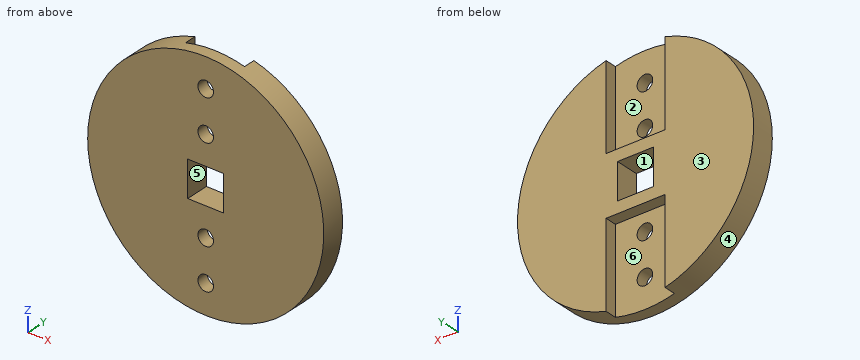
Autodesk Inventor part; units mm, degrees
ref_plane "Work Plane1" through (0, 0, 20) normal (0, 0, 1) x (1, 0, 0)
ref_plane "YZ Plane" through (0, 0, 0) normal (1, 0, 0) x (0, 1, 0)
ref_plane "XZ Plane" through (0, 0, 0) normal (0, 1, 0) x (-1, 0, 0)
sketch "Sketch1" plane through (0, 0, 0) normal (0, 1, 0) x (-1, 0, 0)
  circle A0 centre (0, 0) radius 20
  dimension "d0" = 40
extrude "Extrusion1" add sketch "Sketch1" along normal blind 6
sketch "Sketch3" plane through (0, 6, 0) normal (0, 1, 0) x (1, 0, 0)
  line L0 (0, 0) -> (0, 20)
  circle A0 centre (0, 0) radius 20
  line L1 (5, 35) -> (5, 5)
  line L2 (5, 5) -> (-5, 5)
  line L3 (-5, 5) -> (-5, 35)
  line L4 (-5, 35) -> (5, 35)
  line L5 (5, 35) -> (-5, 5) construction
  line L6 (5, 5) -> (-5, 35) construction
  line L7 (20, 0) -> (-20, 0) construction
  line L8 (5, -35) -> (5, -5)
  line L9 (5, -5) -> (-5, -5)
  line L10 (-5, -5) -> (-5, -35)
  line L11 (-5, -35) -> (5, -35)
  point P0 (-5, 19.3649)
  point P1 (5, 19.3649)
  point P2 (-5, -19.3649)
  point P3 (5, -19.3649)
  dimension "d11" = 30
  dimension "d12" = 10
extrude "Extrusion2" cut sketch "Sketch3" against normal blind 2 contours L2 L3 A0 L0 | L0 A0 L1 L2 | L10 L9 L8 A0
sketch "Sketch5" plane through (0, 4, 0) normal (0, 1, 0) x (1, 0, 0)
  circle A0 centre (0, -8) radius 1
  circle A1 centre (0, -15) radius 1
  line L0 (-5, -5) -> (5, -5)
  arc A2 (-5, 19.3649) -> (-5, -19.3649) centre (0, 0) ccw
  line L1 (-20, 0) -> (20, 0) construction
  arc A3 (5, -19.3649) -> (5, 19.3649) centre (0, 0) ccw
  circle A4 centre (0, 8) radius 1
  circle A5 centre (0, 15) radius 1
  line L2 (-28, 0) -> (28, 0)
  line L3 (-5, 5) -> (-5, 19.3649)
  dimension "d20" = 2
  dimension "d21" = 2
  dimension "d42" = 8
  dimension "d43" = 7
  dimension "d44" = 8
  dimension "d45" = 20
  dimension "d47" = 5
hole "Hole2" at (0, 4, 15) at (0, 4, 8) at (0, 4, -8) at (0, 4, -15) direction (0, -1, 0) diameter 2.6416 depth 10.979 tip angle 118
sketch "Sketch6" plane through (0, 6, 0) normal (0, 1, 0) x (1, 0, 0)
  line L0 (3.05, 3.05) -> (-3.05, 3.05)
  line L1 (-3.05, 3.05) -> (-3.05, -3.05)
  line L2 (-3.05, -3.05) -> (3.05, -3.05)
  line L3 (3.05, -3.05) -> (3.05, 3.05)
  point P0 (0, 0)
  dimension "d31" = 6.1
  dimension "d32" = 6.1
  dimension "d33" = 3.05
  dimension "d34" = 3.05
extrude "Extrusion4" cut sketch "Sketch6" against normal blind 10
ref_plane "Work Plane1" through (0, 0, 20) normal (0, 0, 1) x (1, 0, 0)
sketch "Sketch7" plane through (0, 0, 20) normal (0, 0, 1) x (1, 0, 0)
  line L0 (20, 0) -> (-20, 0)
  line L1 (-20, 0) -> (20, 0)
  line L2 (20, 0) -> (20, 2)
  line L3 (20, 2) -> (-20, 2)
  line L4 (-20, 2) -> (-20, 0)
  point P0 (0, 0)
  dimension "d38" = 40
  dimension "d39" = 2
extrude "Extrusion5" cut sketch "Sketch7" against normal blind 40
sketch "Sketch8" plane through (0, 6, 0) normal (0, 1, 0) x (1, 0, 0)
  line L0 (-20, -20) -> (-7, -20)
  line L1 (-7, -20) -> (-7, 20)
  line L2 (-7, 20) -> (-20, 20)
  line L3 (-20, 20) -> (-20, -20)
  line L4 (7, -20) -> (20, -20)
  line L5 (20, -20) -> (20, 20)
  line L6 (20, 20) -> (7, 20)
  line L7 (7, 20) -> (7, -20)
  line L8 (5, 19.3649) -> (5, 5)
  line L9 (-5, 5) -> (-5, 19.3649)
  line L10 (28.233, -20) -> (-28.0388, -20)
  point P0 (0, 0)
  dimension "d48" = 40
  dimension "d49" = 0
  dimension "d50" = 0
  dimension "d51" = 2
  dimension "d52" = 2
  dimension "d53" = 0
  dimension "d54" = 13
  dimension "d55" = 13
properties part number "prop_base"
Can you work these out from the model? Positions are in its coordinate system, mm. Face numbers are marked on the shaded views. A direction names the side the tool comes from. Round coordinates to 2 decimals unless told otherwise and drop trailing zeros. Loops run counter-clockwise (first coordinate to the right, second up) from the corner with the lowest first, then second, coordinate; pieces in that order, holes last. Notation, with made-up numbers: M 67.25,20 L 111.25,20 A22 cw 111.25,39 Z; hole C 24,67.25 d10. An arc over 180 degrees is marked long. Answer as a JSON object with one key per item and string values. Group by question number.
Q1. Will these pins go through, and if not, where does the flat tip stop? pin 1 (1 mm diameter, centred on y = 5.5, z = -3.5, fed in from -X); pin 2 (2 mm diameter, centred on y = 5.5, z = 14.5, fed in from +X); pin 3 (1 mm diameter, centred on y = 5, z = -10, fed in from +X); pin 4 (1.6 mm diameter, centred on x = 0, z = 8, fed in from +Y).
Q2. On a 3-axis mill with a long thin cutter (end or side, diameter ignored), from which of +Z, -Z, +X, -X, +Y, -Y can I reach the whole of each face in a straight line? I mean the marked faces 1, 2 and 3. Say none if no direction works.
Q3. We'd pull the mould along Z, two halves only. Please class the marked faces 4, 5 and 6: +Z half, -Z half, draft (parallel to the pull), parting line (faces both ways), or undercut.
Q4. Imagine slicing it at C-C, the plane x = 0. Please give me the cut outline in (y, z).
Q5. Imagine slicing it at B-B, the plane z = 0. Please give me the cut outline in (x, y), then the cut area to 3 significant figures.
Q6. Imagine slicing it at D-D, the plane z = -6. Please give me the cut outline in (x, y), then the cut area to 3 significant figures.
Q7. Imagine slicing it at A-A, the plane y = 4.7. Please give me the cut outline in (x, z), then the cut area to 3 significant figures.
Q8. Please list where these lines run through material, in increasing order: L1, parallel to Z at x = 0, y = 2.8; L2, parallel to Z at x = 0.5, y = 2.2; L3, parallel to X at y = 2.9, z = -8.
Findings:
{
 "1": {"pin 1": "stops at x = -19.77", "pin 2": "stops at x = 14.76", "pin 3": "stops at x = 17.6", "pin 4": "passes through"},
 "2": {"face 1": "+Y, -Y", "face 2": "+Z, +Y", "face 3": "+Z, -Z, +X, -X, +Y"},
 "3": {"face 4": "parting line", "face 5": "undercut", "face 6": "draft"},
 "4": {"outline": "M 2,-20 L 4,-20 L 4,-16.32 L 2,-16.32 Z; M 2,-13.68 L 4,-13.68 L 4,-9.32 L 2,-9.32 Z; M 2,-6.68 L 4,-6.68 L 4,-5 L 6,-5 L 6,-3.05 L 2,-3.05 Z; M 2,3.05 L 6,3.05 L 6,5 L 4,5 L 4,6.68 L 2,6.68 Z; M 2,9.32 L 4,9.32 L 4,13.68 L 2,13.68 Z; M 2,16.32 L 4,16.32 L 4,20 L 2,20 Z"},
 "5": {"outline": "M -20,2 L -3.05,2 L -3.05,6 L -20,6 Z; M 3.05,2 L 20,2 L 20,6 L 3.05,6 Z", "area": "136 mm2"},
 "6": {"outline": "M -19.08,2 L 19.08,2 L 19.08,6 L 5,6 L 5,4 L -5,4 L -5,6 L -19.08,6 Z", "area": "133 mm2"},
 "7": {"outline": "M -5,-19.36 L -5,-5 L 5,-5 L 5,-19.36 A20 ccw 5,19.36 L 5,5 L -5,5 L -5,19.36 A20 ccw Z; hole M -3.05,-3.05 L 3.05,-3.05 L 3.05,3.05 L -3.05,3.05 Z", "area": "924 mm2"},
 "8": {"L1": "z = -20 to -16.32, -13.68 to -9.32, -6.68 to -3.05, 3.05 to 6.68, 9.32 to 13.68, 16.32 to 20", "L2": "z = -19.99 to -16.22, -13.78 to -9.22, -6.78 to -3.05, 3.05 to 6.78, 9.22 to 13.78, 16.22 to 19.99", "L3": "x = -18.33 to -1.32, 1.32 to 18.33"}
}
